from build123d import *

# Parameters (mm, degrees)
SKETCH1_R           = 30
SKETCH1_R_2         = 7
BOSS_EXTRUDE1_DEPTH = 10
CUT_EXTRUDE1_DEPTH  = 9
CUT_EXTRUDE2_DEPTH  = 12


with BuildPart() as part:
    # Sketch1 → Boss-Extrude1 (new body, symmetric)
    with BuildSketch(Plane.XY):
        with BuildLine():
            Line((128.063755469, 9.084385863), (27.935473676, 25.760615491))
            ThreePointArc((27.935473676, 25.760615491), (-38, 0), (27.935473676, -25.760615491))
            Line((27.935473676, -25.760615491), (128.063755469, -9.084385863))
            ThreePointArc((128.063755469, -9.084385863), (155, 0), (128.063755469, 9.084385863))
        make_face()
        Circle(SKETCH1_R, mode=Mode.SUBTRACT)
        with Locations((140, 0)):
            Circle(SKETCH1_R_2, mode=Mode.SUBTRACT)
    extrude(amount=BOSS_EXTRUDE1_DEPTH, both=True)

    # Sketch2 → Cut-Extrude1 (cut)
    with BuildSketch(Plane.XY.offset(10)):
        with BuildLine():
            Line((41.828554558, 17.870982725), (122.478416149, 4.438857582))
            ThreePointArc((122.478416149, 4.438857582), (126.239130435, 0), (122.478416149, -4.438857582))
            Line((122.478416149, -4.438857582), (41.828554558, -17.870982725))
            ThreePointArc((41.828554558, -17.870982725), (37.231968897, -16.217361812), (36.238855523, -11.43439331))
            ThreePointArc((36.238855523, -11.43439331), (38, 0), (36.238855523, 11.43439331))
            ThreePointArc((36.238855523, 11.43439331), (37.231968897, 16.217361812), (41.828554558, 17.870982725))
        make_face()
    cut_extrude1 = extrude(amount=-CUT_EXTRUDE1_DEPTH, mode=Mode.SUBTRACT)

    # Mirror1: Cut-Extrude1 across plane
    add(cut_extrude1.mirror(Plane.XY), mode=Mode.SUBTRACT)

    # Sketch3 → Cut-Extrude2 (cut, through all)
    with BuildSketch(Plane.XY.offset(1)):
        with BuildLine():
            Line((47.517939236, -6.785679827), (88.260869565, 0))
            Line((88.260869565, 0), (47.517939236, 6.785679827))
            ThreePointArc((47.517939236, 6.785679827), (48, 0), (47.517939236, -6.785679827))
        make_face()
    extrude(amount=-CUT_EXTRUDE2_DEPTH, mode=Mode.SUBTRACT)


solid = part.part
Here's how the part is built. I have some questions about the finished solid (model axes, mm). A direction names the side the tool comes from. Round coordinates to 2 decimals unless told otherwise and drop trailing zeros. Write each loop counter-clockwise with the first axis right and the second up, starting at its lowest first coordinate (ties: lowest second). Pieces come first, ordered by that corner, then holes.
1. Suppose I cut it at B-B (z = -8). List the corners of the cut face in (x, y) for me, and give its area (3 significant figures).
2. Suppose I cut it at D-D (x = 104.5). List the corners of the cut face in (y, z) for me, and give its area (3 significant figures).
3. Suppose I cut it at C-C (y = -23.5). List the corners of the cut face in (x, z) for me.
4. I need wall thicknesses on L1, parallel to X at y = -1.5, z = -5; L2, parallel to Z at x = 70.5, y = -8; L3, parallel to Y at x = 43.5, z = 8.25. Which ranges of each line are inside material? Lowest first, please.
5. For faces 1 (the cylindrical face through (37.186, 16.163, 5.563)), 2 (the flat face through (37, 0, 10)), 3 (the cylindrical face through (37.186, 16.163, -5.563)), 4 (the flat face through (67.6, -3.44, 0.01)), which set-ups out of +Z, -Z, +X, -X, +Y, -Y let a thin tool reach every point of the face, with its end or its side?
6. If we mould it in two halves opening along Y, with no side actions, what happens to faces 5 (the flat face through (68.175, 3.345, 0.014)), 6 (the flat face through (78.701, 17.306, 0.14)), 7 (the cylindrical face through (154.99, -0.52, 0.14))? For each: released by +Y, released by -Y, zero draft, split by the parting line, or undercut.
7. Will these pins go through, and if not, where does the flat tip stop? pin 1 Ø4 at (y, z) = (2.5, -4.5) entering from +X; pin 2 Ø12 at (x, z) = (38.5, 2) entering from -Y; pin 3 Ø1.5 at (y, z) = (-23, -2.5) entering from -X; pin 4 Ø12.5 at (x, y) = (140, 0) entering from -Z.
8. Suppose I cut it at A-A (x = 0). List the corners of the cut face in (y, z) for me.
Answer sheet:
1. outline: (27.94, -25.76) - (128.06, -9.08) arc R15 ccw (long way) to (128.06, 9.08) - (27.94, 25.76) arc R38 ccw (long way) to start; hole circle Ø60 at (0, 0); hole (36.24, -11.43) arc R5 ccw to (41.83, -17.87) - (122.48, -4.44) arc R4.5 ccw to (122.48, 4.44) - (41.83, 17.87) arc R5 ccw to (36.24, 11.43) arc R38 cw to start; hole circle Ø14 at (140, 0)
1. area: 3,370 mm2
2. outline: (-13.01, -10) - (-7.43, -10) - (-7.43, -1) - (7.43, -1) - (7.43, -10) - (13.01, -10) - (13.01, 10) - (7.43, 10) - (7.43, 1) - (-7.43, 1) - (-7.43, 10) - (-13.01, 10) - close
2. area: 253 mm2
3. outline: (-29.86, -10) - (-18.65, -10) - (-18.65, 10) - (-29.86, 10) - close; (18.65, -10) - (41.51, -10) - (41.51, 10) - (18.65, 10) - close
4. L1: x = -37.97 to -29.96, 29.96 to 37.97, 125.98 to 133.16, 146.84 to 154.92
4. L2: z = -1 to 1
4. L3: y = -23.17 to -17.59, 17.59 to 23.17
5. face 1: +Z
5. face 2: +Z, +X, -X, +Y, -Y
5. face 3: -Z
5. face 4: +Z, -Z
6. face 5: undercut
6. face 6: released by +Y
6. face 7: split by the parting line
7. pin 1: stops at x = 154.99
7. pin 2: stops at y = -25
7. pin 3: stops at x = -30.8
7. pin 4: passes through
8. outline: (-38, -10) - (-30, -10) - (-30, 10) - (-38, 10) - close; (30, -10) - (38, -10) - (38, 10) - (30, 10) - close
